The listing builds one solid part. Answer for the finished solid, in the listing's coordinates (mm). Face numbers are marked on the shaded views. A direction names the side the tool comes from. Coordinates: 2 decimals unless noted, no trailing zeros. Order: outer loops, then holes, each group sorted by start corner. A loop starts at its lowest first (then second) coordinate and runs counter-clockwise, first axis right, second up. Notation, with made-up numbers: M 18,34 L 35,34 A27 ccw 35,63 Z; hole C -16.5,32.5 d5. An arc over 180 degrees is marked long. One line per item, written item: value. Start each with the question number.
Q1. For the marked faces 4, 5 and 6, determine the directions among +Z, -Z, +X, -X, +Y, -Y from which every point of the face is accessible in a straight line to the end or side of a thin tool.
Q2. Straight lines are drawn through the part: line 1 along Y through (x, z) = (7.25, 3.5); line 2 along Y through (x, z) = (-0.25, 1.3). For each, find the intervals that lie inside material, in ascending order. Write a range as [from, to].
Q3. The part is cut by section D-D on y = 6.65. Give the vertices of the cut face in (x, z), then the cut area to 3 significant figures.
Q4. Determine the mould class of the marked faces 1, 2 and 3 for opening direction X: pulls with the +X half, pulls with the -X half, needs draft (parallel to the pull), parting line crosses it, or undercut.
Q5. The part is cut by section A-A on y = 5.8. Give the vertices of the cut face in (x, z), then the cut area to 3 significant figures.
Q6. The part is cut by section C-C on x = 4.25. Give the vertices of the cut face in (y, z), then the cut area to 3 significant figures.
Q7. This flat-tipped pin is pushed along its axis until it touches: pin 1 Ø1 at (x, z) = (-4, 4) entering from -Y. Where does it stop, or does it pass through?
Autodesk Inventor part; units mm, degrees
ref_plane "YZ Plane" through (0, 0, 0) normal (1, 0, 0) x (0, 1, 0)
ref_plane "XZ Plane" through (0, 0, 0) normal (0, 1, 0) x (-1, 0, 0)
ref_plane "XY Plane" through (0, 0, 0) normal (0, 0, 1) x (1, 0, 0)
sketch "Sketch1" plane through (0, 0, 0) normal (0, 0, 1) x (1, 0, 0)
  line L0 (0, -9.4281) -> (0, 9.3187)
  arc A0 (6.7496, 0.073) -> (6.51, 0.4187) centre (6.3746, 0.0689) ccw
  arc A1 (-6.7496, 0.073) -> (6.7496, 0.073) centre (0, 0) ccw
  arc A2 (-6.51, 0.4187) -> (-6.7496, 0.073) centre (-6.3746, 0.0689) ccw
  arc A3 (-4.3687, 0.6769) -> (-6.51, 0.4187) centre (-4.9321, -3.658) ccw
  arc A4 (-4.3687, 0.6769) -> (-4.2435, 0.7684) centre (-4.3542, 0.7885) ccw
  arc A5 (-4.2145, 0.914) -> (-4.2435, 0.7684) centre (0, 0) ccw
  arc A6 (-4.2145, 0.914) -> (-4.2952, 1.0464) centre (-4.3245, 0.9378) ccw
  arc A7 (-6.1747, 2.1045) -> (-4.2952, 1.0464) centre (-3.1568, 5.267) ccw
  arc A8 (-6.2638, 2.5155) -> (-6.1747, 2.1045) centre (-5.9158, 2.3758) ccw
  arc A9 (-6.0212, 3.0507) -> (-6.2638, 2.5155) centre (0, 0) ccw
  arc A10 (-5.6535, 3.2548) -> (-6.0212, 3.0507) centre (-5.6867, 2.8813) ccw
  arc A11 (-3.6188, 2.5393) -> (-5.6535, 3.2548) centre (-6.0413, -1.0993) ccw
  arc A12 (-3.6188, 2.5393) -> (-3.466, 2.566) centre (-3.5564, 2.633) ccw
  arc A13 (-3.3757, 2.6838) -> (-3.466, 2.566) centre (0, 0) ccw
  arc A14 (-3.3757, 2.6838) -> (-3.3894, 2.8382) centre (-3.4637, 2.7538) ccw
  arc A15 (-4.6071, 4.6184) -> (-3.3894, 2.8382) centre (-0.5017, 6.12) ccw
  arc A16 (-4.5052, 5.0265) -> (-4.6071, 4.6184) centre (-4.2549, 4.7472) ccw
  arc A17 (-4.051, 5.3993) -> (-4.5052, 5.0265) centre (0, 0) ccw
  arc A18 (-3.6309, 5.4196) -> (-4.051, 5.3993) centre (-3.8259, 5.0993) ccw
  arc A19 (-2.1225, 3.878) -> (-3.6309, 5.4196) centre (-5.9045, 1.6861) ccw
  arc A20 (-2.1225, 3.878) -> (-1.9736, 3.8344) centre (-2.0251, 3.9344) ccw
  arc A21 (-1.8405, 3.9) -> (-1.9736, 3.8344) centre (0, 0) ccw
  arc A22 (-1.8405, 3.9) -> (-1.7845, 4.0446) centre (-1.8886, 4.0017) ccw
  arc A23 (-2.0893, 6.1798) -> (-1.7845, 4.0446) centre (2.2568, 5.7108) ccw
  arc A24 (-1.8174, 6.5007) -> (-2.0893, 6.1798) centre (-1.7165, 6.1396) ccw
  arc A25 (-1.2452, 6.6342) -> (-1.8174, 6.5007) centre (0, 0) ccw
  arc A26 (-0.8594, 6.4666) -> (-1.2452, 6.6342) centre (-1.176, 6.2656) ccw
  arc A27 (-0.1884, 4.4168) -> (-0.8594, 6.4666) centre (-4.5499, 4.1237) ccw
  arc A28 (-0.1884, 4.4168) -> (-0.0742, 4.3119) centre (-0.0761, 4.4243) ccw
  arc A29 (0.0742, 4.3119) -> (-0.0742, 4.3119) centre (0, 0) ccw
  arc A30 (0.0742, 4.3119) -> (0.1884, 4.4168) centre (0.0761, 4.4243) ccw
  arc A31 (0.8594, 6.4666) -> (0.1884, 4.4168) centre (4.5499, 4.1237) ccw
  arc A32 (1.2452, 6.6342) -> (0.8594, 6.4666) centre (1.176, 6.2656) ccw
  arc A33 (1.8174, 6.5007) -> (1.2452, 6.6342) centre (0, 0) ccw
  arc A34 (2.0893, 6.1798) -> (1.8174, 6.5007) centre (1.7165, 6.1396) ccw
  arc A35 (1.7845, 4.0446) -> (2.0893, 6.1798) centre (-2.2568, 5.7108) ccw
  arc A36 (1.7845, 4.0446) -> (1.8405, 3.9) centre (1.8886, 4.0017) ccw
  arc A37 (1.9736, 3.8344) -> (1.8405, 3.9) centre (0, 0) ccw
  arc A38 (1.9736, 3.8344) -> (2.1225, 3.878) centre (2.0251, 3.9344) ccw
  arc A39 (3.6309, 5.4196) -> (2.1225, 3.878) centre (5.9045, 1.6861) ccw
  arc A40 (4.051, 5.3993) -> (3.6309, 5.4196) centre (3.8259, 5.0993) ccw
  arc A41 (4.5052, 5.0265) -> (4.051, 5.3993) centre (0, 0) ccw
  arc A42 (4.6071, 4.6184) -> (4.5052, 5.0265) centre (4.2549, 4.7472) ccw
  arc A43 (3.3894, 2.8382) -> (4.6071, 4.6184) centre (0.5017, 6.12) ccw
  arc A44 (3.3894, 2.8382) -> (3.3757, 2.6838) centre (3.4637, 2.7538) ccw
  arc A45 (3.466, 2.566) -> (3.3757, 2.6838) centre (0, 0) ccw
  arc A46 (3.466, 2.566) -> (3.6188, 2.5393) centre (3.5564, 2.633) ccw
  arc A47 (5.6535, 3.2548) -> (3.6188, 2.5393) centre (6.0413, -1.0993) ccw
  arc A48 (6.0212, 3.0507) -> (5.6535, 3.2548) centre (5.6867, 2.8813) ccw
  arc A49 (6.2638, 2.5155) -> (6.0212, 3.0507) centre (0, 0) ccw
  arc A50 (6.1747, 2.1045) -> (6.2638, 2.5155) centre (5.9158, 2.3758) ccw
  arc A51 (4.2952, 1.0464) -> (6.1747, 2.1045) centre (3.1568, 5.267) ccw
  arc A52 (4.2952, 1.0464) -> (4.2145, 0.914) centre (4.3245, 0.9378) ccw
  arc A53 (4.2435, 0.7684) -> (4.2145, 0.914) centre (0, 0) ccw
  arc A54 (4.2435, 0.7684) -> (4.3687, 0.6769) centre (4.3542, 0.7885) ccw
  arc A55 (6.51, 0.4187) -> (4.3687, 0.6769) centre (4.9321, -3.658) ccw
  circle A56 centre (0, 0) radius 1.5
  line L1 (-10, 6.8906) -> (10, 6.8906)
  line L2 (-10, 6.8906) -> (-10, 7.8906)
  line L3 (-10, 7.8906) -> (10, 7.8906)
  line L4 (10, 7.8906) -> (10, 6.8906)
  line L5 (-10, 6.6406) -> (10, 6.6406) construction
  line L6 (0, 4.7099) -> (-1.3614, 7.6295) construction
  line L7 (-0.5881, 5.9711) -> (0.5881, 5.9711) construction
  line L8 (-1.4832, 7.8906) -> (0, 4.7099) construction
  line L9 (0.5881, 5.9711) -> (-0.5881, 5.9711) construction
  arc A57 (-0.7, 6.8906) -> (-0.1371, 5.2406) centre (7.2211, 8.6718) ccw
  line L10 (-0.1371, 5.2406) -> (0.1371, 5.2406)
  arc A58 (0.1371, 5.2406) -> (0.7, 6.8906) centre (-7.2211, 8.6718) ccw
  line L11 (-1.3728, 7.8906) -> (0, 4.9465) construction
  point P0 (0, 6.8906)
  dimension "d0" = 20
  dimension "d1" = 0.25
  dimension "d2" = 1
  dimension "d3" = 0.1
  dimension "d4" = 1.4
  dimension "d5" = 1.65
extrude "Extrusion1" add sketch "Sketch1" along normal blind 6 contours L10 A57 L1 L0 | L0 L1 A58 L10
sketch "Sketch3" plane through (0, 0, 0) normal (0, 0, 1) x (1, 0, 0)
  line L0 (-10, 7.8906) -> (10, 7.8906)
  line L1 (-10, 6.8906) -> (-10, 7.8906)
  line L2 (-10, 6.8906) -> (10, 6.8906)
  line L3 (10, 7.8906) -> (10, 6.8906)
  point P0 (0, 0)
extrude "Extrusion2" add sketch "Sketch3" along normal up to surface (6 mm away)
pattern_linear "Rectangular Pattern1" count 7 spacing 2.7 along (1, 0, 0) of "Extrusion1" first direction both ways yes
equation "\"d12\" = 3.6 * model_gear_module"
properties part number "rack_test"
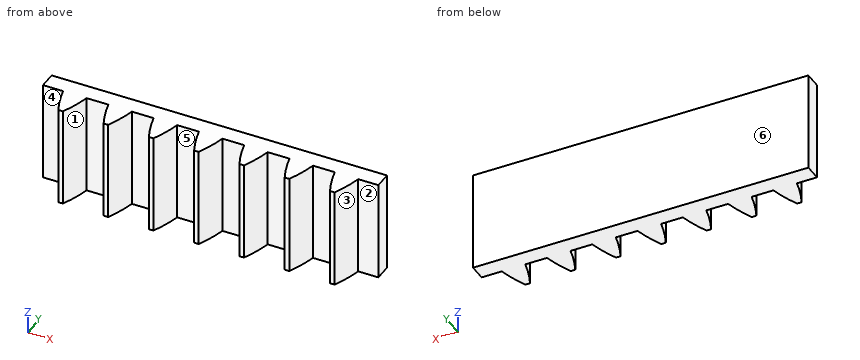
Output:
1. face 4: +Z, -Z, -X, -Y
1. face 5: +Z, -Z, -Y
1. face 6: +Z, -Z, +X, -X, +Y
2. line 1: y = [6.89, 7.89]
2. line 2: y = [5.49, 7.89]
3. outline: M -8.74,0 L -7.46,0 L -7.46,6 L -8.74,6 Z; M -6.04,0 L -4.76,0 L -4.76,6 L -6.04,6 Z; M -3.34,0 L -2.06,0 L -2.06,6 L -3.34,6 Z; M -0.64,0 L 0.64,0 L 0.64,6 L -0.64,6 Z; M 2.06,0 L 3.34,0 L 3.34,6 L 2.06,6 Z; M 4.76,0 L 6.04,0 L 6.04,6 L 4.76,6 Z; M 7.46,0 L 8.74,0 L 8.74,6 L 7.46,6 Z
3. area: 53.9 mm^2
4. face 1: undercut
4. face 2: needs draft
4. face 3: pulls with the +X half
5. outline: M -8.47,0 L -7.73,0 L -7.73,6 L -8.47,6 Z; M -5.77,0 L -5.03,0 L -5.03,6 L -5.77,6 Z; M -3.07,0 L -2.33,0 L -2.33,6 L -3.07,6 Z; M -0.37,0 L 0.37,0 L 0.37,6 L -0.37,6 Z; M 2.33,0 L 3.07,0 L 3.07,6 L 2.33,6 Z; M 5.03,0 L 5.77,0 L 5.77,6 L 5.03,6 Z; M 7.73,0 L 8.47,0 L 8.47,6 L 7.73,6 Z
5. area: 31.3 mm^2
6. outline: M 6.89,0 L 7.89,0 L 7.89,6 L 6.89,6 Z
6. area: 6.00 mm^2
7. pin 1: stops at y = 6.89
